Can you work these out from the model? Positions are in its coordinate system, mm. A direction names the side the tool comes from. Give positions to 0.01 mm unless a question says otherwise; leave off trailing zeros. Loops run counter-clockwise (first coordinate to the right, second up) from the corner with the lowest first, then second, coordinate; pieces in that order, holes last. Notation, with made-up numbers: M 82,1 L 139,1 A26 ccw 139,33 Z; hole C -14,-36.75 d4. An arc over 180 degrees is marked long. Answer as a JSON object with one key per item and string values.
```python
from build123d import *

# Parameters (mm, degrees)
SKETCH1_R           = 2
BOSS_EXTRUDE1_DEPTH = 2


with BuildPart() as part:
    # Sketch1 → Boss-Extrude1 (new body)
    with BuildSketch(Plane.XY):
        with BuildLine():
            Line((10.224721825, -6.524941173), (10.088449683, 4.475058827))
            Line((10.088449683, 4.475058827), (25.088449683, 4.475058827))
            Line((25.088449683, 4.475058827), (25.088449683, 12.475058827))
            Line((25.088449683, 12.475058827), (10.027054239, 12.475058827))
            Line((10.027054239, 12.475058827), (10.027054239, 23.2867844))
            ThreePointArc((10.027054239, 23.2867844), (2.527054239, 30.7867844), (-4.972945761, 23.2867844))
            Line((-4.972945761, 23.2867844), (-4.972945761, -6.7132156))
            ThreePointArc((-4.972945761, -6.7132156), (2.627054239, -14.3132156), (10.227054239, -6.7132156))
            Line((10.227054239, -6.7132156), (10.224721825, -6.524941173))
        make_face()
        with Locations((2.627054239, -6.7132156)):
            Circle(SKETCH1_R, mode=Mode.SUBTRACT)
        with Locations((2.527054239, 23.2867844)):
            Circle(SKETCH1_R, mode=Mode.SUBTRACT)
    extrude(amount=BOSS_EXTRUDE1_DEPTH)


solid = part.part
```
1) Suppose I cut it at A-A, the plane y = 22.5. Write out the boundary of the cut face in (x, z).
Answer list:
{"outline": "M -4.97,0 L 0.69,0 L 0.69,2 L -4.97,2 Z; M 4.37,0 L 10.03,0 L 10.03,2 L 4.37,2 Z"}
2) Suppose I cut it at D-D, the plane y = 15. Write out the boundary of the cut face in (x, z).
Answer list:
{"outline": "M -4.97,0 L 10.03,0 L 10.03,2 L -4.97,2 Z"}
3) Will these pins go through, and if not, where does the flat tip stop? pin 1 Ø1 at (x, z) = (11.5, 1) entering from +Y; pin 2 Ø3 at (x, y) = (2.63, -6.71) entering from +Z; pin 3 Ø3 at (x, y) = (13.5, 11.5) entering from -Z.
Answer list:
{"pin 1": "y = 12.48", "pin 2": "through", "pin 3": "z = 0"}
4) Please list where these lines run through material, in increasing order: line 1 along Y through (x, z) = (22, 0.55); line 2 along X through (y, z) = (21, 0.55); line 3 along X through (y, z) = (22, 1.55). Write a range as from..to.
Answer list:
{"line 1": "4.48..12.48", "line 2": "-4.97..10.03", "line 3": "-4.97..1, 4.06..10.03"}
5) If we mould it in two halves opening along X, with no side actions, what happens to faces 3 (the cylindrical face through (2.37, -4.73, 0.99)), 4 (the flat face through (3, 9, 2)), 5 (the cylindrical face through (2.692, 30.785, 0.986)), 6 (the flat face through (-4.973, 8, 1))? For each: +X half, -X half, draft (parallel to the pull), parting line (faces both ways), or undercut.
Answer list:
{"face 3": "undercut", "face 4": "draft", "face 5": "parting line", "face 6": "-X half"}
6) Suppose I cut it at B-B, the plane x = 2.5. Write out the boundary of the cut face in (y, z), and give its area (3 significant figures).
Answer list:
{"outline": "M -14.31,0 L -8.71,0 L -8.71,2 L -14.31,2 Z; M -4.72,0 L 21.29,0 L 21.29,2 L -4.72,2 Z; M 25.29,0 L 30.79,0 L 30.79,2 L 25.29,2 Z", "area": "74.2 mm^2"}
7) Suppose I cut it at C-C, the plane z = 1.55. Write out the boundary of the cut face in (x, y).
Answer list:
{"outline": "M -4.97,-6.71 A7.6 ccw 10.23,-6.71 L 10.09,4.48 L 25.09,4.48 L 25.09,12.48 L 10.03,12.48 L 10.03,23.29 A7.5 ccw -4.97,23.29 Z; hole C 2.53,23.29 d4; hole C 2.63,-6.71 d4"}
8) For faces 1 (the flat face through (10.027, 18, 1)), 2 (the flat face through (3, 9, 0)), which set-ups out of +Z, -Z, +X, -X, +Y, -Y let a thin tool reach every point of the face, with its end or its side?
Answer list:
{"face 1": "+Z, -Z, +X, +Y", "face 2": "-Z, +X, -X, +Y, -Y"}
